```python
from build123d import *

# Parameters (mm, degrees)
BOSS_EXTRUDE1_DEPTH = 150
CUT_EXTRUDE1_REACH  = 210.626
SKETCH2_R           = 3
CUT_EXTRUDE2_REACH  = 210.626
SKETCH3_R           = 3


with BuildPart() as part:
    # Sketch1 → Boss-Extrude1 (new body)
    with BuildSketch(Plane.XY):
        Polygon((0, 0), (0, 105), (105, 105), (105, 100), (5, 100), (5, 0), align=None)
    extrude(amount=BOSS_EXTRUDE1_DEPTH)

    # Sketch2 → Cut-Extrude1 (cut, up to next)
    with BuildSketch(Plane(origin=(5, 0, 0), x_dir=(0, 0, -1), z_dir=(1, 0, 0)), mode=Mode.PRIVATE) as cut_extrude1_sk1:
        with Locations(Location((-135, 85, 0), (0, 0, 90))):
            Circle(SKETCH2_R)
    cut_extrude1_tool1 = extrude(cut_extrude1_sk1.sketch, amount=-CUT_EXTRUDE1_REACH, mode=Mode.PRIVATE) & part.part
    # Sketch2 → Cut-Extrude1 (cut, up to next)
    with BuildSketch(Plane(origin=(5, 0, 0), x_dir=(0, 0, -1), z_dir=(1, 0, 0)), mode=Mode.PRIVATE) as cut_extrude1_sk2:
        with Locations((-15, 85)):
            Circle(SKETCH2_R)
    cut_extrude1_tool2 = extrude(cut_extrude1_sk2.sketch, amount=-CUT_EXTRUDE1_REACH, mode=Mode.PRIVATE) & part.part
    # Sketch2 → Cut-Extrude1 (cut, up to next)
    with BuildSketch(Plane(origin=(5, 0, 0), x_dir=(0, 0, -1), z_dir=(1, 0, 0)), mode=Mode.PRIVATE) as cut_extrude1_sk3:
        with Locations(Location((-15, 15, 0), (0, 0, 90))):
            Circle(SKETCH2_R)
    cut_extrude1_tool3 = extrude(cut_extrude1_sk3.sketch, amount=-CUT_EXTRUDE1_REACH, mode=Mode.PRIVATE) & part.part
    # Sketch2 → Cut-Extrude1 (cut, up to next)
    with BuildSketch(Plane(origin=(5, 0, 0), x_dir=(0, 0, -1), z_dir=(1, 0, 0)), mode=Mode.PRIVATE) as cut_extrude1_sk4:
        with Locations((-135, 15)):
            Circle(SKETCH2_R)
    cut_extrude1_tool4 = extrude(cut_extrude1_sk4.sketch, amount=-CUT_EXTRUDE1_REACH, mode=Mode.PRIVATE) & part.part
    add(cut_extrude1_tool1.solids().sort_by_distance((5, 85, 135))[0], mode=Mode.SUBTRACT)
    add(cut_extrude1_tool2.solids().sort_by_distance((5, 85, 15))[0], mode=Mode.SUBTRACT)
    add(cut_extrude1_tool3.solids().sort_by_distance((5, 15, 15))[0], mode=Mode.SUBTRACT)
    add(cut_extrude1_tool4.solids().sort_by_distance((5, 15, 135))[0], mode=Mode.SUBTRACT)

    # Sketch3 → Cut-Extrude2 (cut, up to next)
    with BuildSketch(Plane.XZ.offset(-100), mode=Mode.PRIVATE) as cut_extrude2_sk1:
        with Locations((35, 105)):
            Circle(SKETCH3_R)
    cut_extrude2_tool1 = extrude(cut_extrude2_sk1.sketch, amount=-CUT_EXTRUDE2_REACH, mode=Mode.PRIVATE) & part.part
    # Sketch3 → Cut-Extrude2 (cut, up to next)
    with BuildSketch(Plane.XZ.offset(-100), mode=Mode.PRIVATE) as cut_extrude2_sk2:
        with Locations((90, 105)):
            Circle(SKETCH3_R)
    cut_extrude2_tool2 = extrude(cut_extrude2_sk2.sketch, amount=-CUT_EXTRUDE2_REACH, mode=Mode.PRIVATE) & part.part
    # Sketch3 → Cut-Extrude2 (cut, up to next)
    with BuildSketch(Plane.XZ.offset(-100), mode=Mode.PRIVATE) as cut_extrude2_sk3:
        with Locations((90, 45)):
            Circle(SKETCH3_R)
    cut_extrude2_tool3 = extrude(cut_extrude2_sk3.sketch, amount=-CUT_EXTRUDE2_REACH, mode=Mode.PRIVATE) & part.part
    # Sketch3 → Cut-Extrude2 (cut, up to next)
    with BuildSketch(Plane.XZ.offset(-100), mode=Mode.PRIVATE) as cut_extrude2_sk4:
        with Locations((35, 45)):
            Circle(SKETCH3_R)
    cut_extrude2_tool4 = extrude(cut_extrude2_sk4.sketch, amount=-CUT_EXTRUDE2_REACH, mode=Mode.PRIVATE) & part.part
    add(cut_extrude2_tool1.solids().sort_by_distance((35, 100, 105))[0], mode=Mode.SUBTRACT)
    add(cut_extrude2_tool2.solids().sort_by_distance((90, 100, 105))[0], mode=Mode.SUBTRACT)
    add(cut_extrude2_tool3.solids().sort_by_distance((90, 100, 45))[0], mode=Mode.SUBTRACT)
    add(cut_extrude2_tool4.solids().sort_by_distance((35, 100, 45))[0], mode=Mode.SUBTRACT)


solid = part.part
```
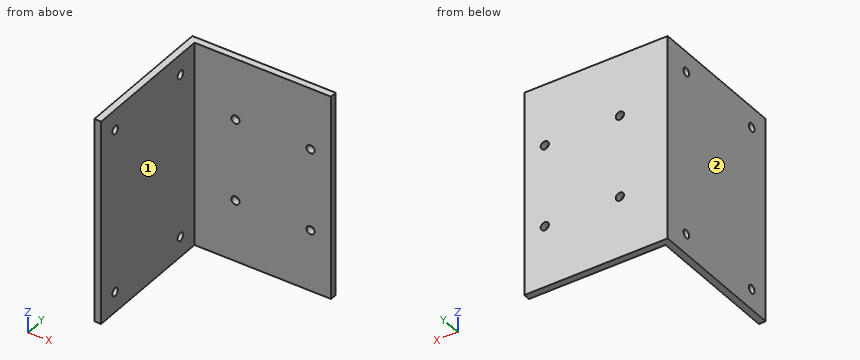
Here's how the part is built. I have some questions about the finished solid (model axes, mm). Face numbers are marked on the shaded views. A direction names the side the tool comes from. Coordinates: 2 decimals unless noted, no trailing zeros. Loops run counter-clockwise (first coordinate to the right, second up) from the corner with the lowest first, then second, coordinate; pieces in that order, holes last. Notation, with made-up numbers: (-38.75, 78) - (6.25, 78) arc R14 cw to (6.25, 101) - close; hole circle Ø7 at (78.5, 16). An arc over 180 degrees is marked (long way). Return JSON: item names as keys, results as strings. Group by question number.
Item 1: If we section it at C-C on x = 35: Write out the boundary of the cut face in (y, z), and give its area (3 significant figures).
Item 2: If we section it at B-B on z = 15: Write out the boundary of the cut face in (x, y), and give its area (3 significant figures).
Item 3: I need wall thicknesses on line 1 (Z direction, x = 90, y = 102.55); line 2 (Y direction, x = 1.6, z = 135); line 3 (Y direction, x = 38, z = 50). Which ranges of each line are inside material? Lowest first, please. Write a range as from..to.
Item 4: If we section it at A-A on y = 85: Write out the boundary of the cut face in (x, z).
Item 5: On a 3-axis mill with a long thin cutter (end or side, diameter ignored), from which of +Z, -Z, +X, -X, +Y, -Y can I reach the whole of each face in a straight line? I mean the marked faces 1 and 2. Say none if no direction works.
Item 6: If we section it at D-D on z = 87: Write out the boundary of the cut face in (x, y), and give its area (4 significant figures).
Item 7: Will these pins go through, and if not, where does the flat tip stop? P1, Ø12, axis at x = 66.5, z = 82.5, coming from the -Y side; P2, Ø5, axis at y = 15, z = 15, coming from the -X side; P3, Ø9.5, axis at y = 85, z = 135, coming from the +X side.
Calculated:
{
 "1": {"outline": "(100, 0) - (105, 0) - (105, 42) - (100, 42) - close; (100, 48) - (105, 48) - (105, 102) - (100, 102) - close; (100, 108) - (105, 108) - (105, 150) - (100, 150) - close", "area": "690 mm^2"},
 "2": {"outline": "(0, 0) - (5, 0) - (5, 12) - (0, 12) - close; (0, 18) - (5, 18) - (5, 82) - (0, 82) - close; (0, 88) - (5, 88) - (5, 100) - (105, 100) - (105, 105) - (0, 105) - close", "area": "965 mm^2"},
 "3": {"line 1": "z = 0..42, 48..102, 108..150", "line 2": "y = 0..12, 18..82, 88..105", "line 3": "y = 100..105"},
 "4": {"outline": "(0, 0) - (5, 0) - (5, 12) - (0, 12) - close; (0, 18) - (5, 18) - (5, 132) - (0, 132) - close; (0, 138) - (5, 138) - (5, 150) - (0, 150) - close"},
 "5": {"face 1": "+Z, -Z, +X, -Y", "face 2": "+Z, -Z, -X, +Y, -Y"},
 "6": {"outline": "(0, 0) - (5, 0) - (5, 100) - (105, 100) - (105, 105) - (0, 105) - close", "area": "1,025 mm^2"},
 "7": {"P1": "stops at y = 100", "P2": "passes through", "P3": "stops at x = 5"}
}
